Could you check a few things on this model? Use its own coordinates, in mm. Face numbers are marked on the shaded views. A direction names the side the tool comes from. Coordinates: 2 decimals unless noted, no trailing zeros. Write each loop counter-clockwise with the first axis right and the second up, starting at its lowest first coordinate (ties: lowest second). Pieces come first, ordered by that corner, then holes. Notation, with made-up numbers: M 88,20.5 L 102,20.5 A35 ccw 102,52.5 Z; hole C -32,54.25 d11. An arc over 180 degrees is marked long. Answer as CSV lines item,"result". Start each with the question number.
Item 1: If I drill on line 1 along Y through (x, z) = (31.5, -0.25); line 2 along X through (y, z) = (-2.5, 2.75); line 3 along Z through (x, y) = (22.5, 0) (3 decimals), over which ranges is the centre line in solid material (lowest first)? Write a range as [from, to].
Item 2: I'm going to push flat-ended pins straight in: P1, Ø1.5, axis at x = 23, z = 0.5, coming from the -Y side (3 decimals); P2, Ø1, axis at x = 1.5, y = 2.5, coming from the -Z side; P3, Ø2, axis at x = 3.5, z = -2, coming from the -Y side. Where does each tip first touch, or does it pass through?
Item 3: Suppose I cut it at A-A, the plane x = 2. Write out the boundary of the cut face in (y, z) (3 decimals), and give its area (3 significant figures).
Item 4: On a 3-axis mill with a long thin cutter (end or side, diameter ignored), from which of +Z, -Z, +X, -X, +Y, -Y can I reach the whole of each face in a straight line? I mean the marked faces 1, 2 and 3. Say none if no direction works.
Autodesk Inventor part; units mm, degrees
ref_plane "Work Plane1" through (29, 0, 0) normal (0, -1, 0) x (1, 0, 0)
ref_plane "YZ Plane" through (0, 0, 0) normal (1, 0, 0) x (0, 1, 0)
ref_plane "XZ Plane" through (0, 0, 0) normal (0, 1, 0) x (-1, 0, 0)
sketch "Sketch1" plane through (0, 0, 0) normal (0, 0, 1) x (1, 0, 0)
  line L0 (-1.7103, 0) -> (50.8, 0)
  line L1 (50.8, 0) -> (50.8, 3.175)
  line L2 (50.8, 3.175) -> (19.05, 3.175)
  line L3 (19.05, 3.175) -> (15.8749, 3.175)
  line L4 (15.8749, 3.175) -> (0, 3.175)
  line L5 (0, 3.175) -> (0, 4.7625)
  line L6 (0, 4.7625) -> (-6.35, 4.7625)
  line L7 (-6.35, 4.7625) -> (-6.35, 2.757)
  line L8 (-6.35, 2.757) -> (-3.302, 2.757)
  line L9 (-3.302, 2.757) -> (-1.7103, 0)
  line L10 (-16.51, 0) -> (54.61, 0)
  line L11 (0, -0.9525) -> (0, 5.715)
  line L12 (19.05, 3.175) -> (0, 3.175) construction
  dimension "d1" = 31.75
  dimension "d2" = 3.1751
  dimension "d3" = 6.35
  dimension "d4" = 3.048
  dimension "d5" = 60
  dimension "d6" = 6.35
  dimension "d7" = 6.35
  dimension "d8" = 5.5139
  dimension "d9" = 9.525
  dimension "d26" = 50.8
revolve "Body" add sketch "Sketch1" angle 360 about axis through (-1.7103, 0, 0) along (1, 0, 0)
sketch "Sketch2" plane through (-6.35, 0, 0) normal (-1, 0, 0) x (0, 0, 1)
  circle A0 centre (0, 0) radius 2.757
  line L0 (0, -6.6675) -> (0, 6.6675)
  line L1 (-6.6675, 0) -> (6.6675, 0)
  line L2 (2.757, 0) -> (1.3785, -2.3876)
  line L3 (1.3785, -2.3876) -> (-1.3785, -2.3876)
  line L4 (-1.3785, -2.3876) -> (-2.757, 0)
  line L5 (-2.757, 0) -> (-1.3785, 2.3876)
  line L6 (-1.3785, 2.3876) -> (1.3785, 2.3876)
  line L7 (1.3785, 2.3876) -> (2.757, 0)
extrude "Slot" add sketch "Sketch2" against normal up to next contours L7 A0 | A0 L2 | L6 L0 A0 | A0 L0 L3 | L0 L6 A0 | A0 L3 L0 | L4 A0 | A0 L5
fillet "Fillet1" radius 0.635 1 edges at (-6.35, -4.7625, 0)
thread "Thread"
chamfer "Chamfer1" distance 0.7556 distance2 0.7556 1 edges at (50.8, -3.175, 0) measured on face at (50.8, -0.8017, -1.6073)
ref_plane "Work Plane1" through (29, 0, 0) normal (0, -1, 0) x (1, 0, 0)
equation "\"d1\" = GEL"
equation "\"d3\" = KOH"
equation "\"d4\" = INTI"
equation "\"d6\" = GD"
equation "\"d7\" = BDM"
equation "\"d8\" = 1.1547 * SW"
equation "\"d9\" = KOD"
equation "\"d26\" = NLG"
equation "\"d17\" = RR"
equation "\"d13\" = GEL"
equation "\"d15\" = -0.5 * SPD + 0.5 * GD"
equation "\"d16\" = GUL"
equation "\"GD\" = 6.35"
equation "\"NLG\" = 50.8"
equation "\"GEL\" = 31.75"
equation "\"KOD\" = 9.525"
equation "\"KOH\" = 6.35"
equation "\"INTI\" = 3.048"
equation "\"GAL\" = 3.175"
equation "\"GUL\" = 0.75565"
equation "\"BDM\" = 6.35"
equation "\"SW\" = 4.7752"
equation "\"RR\" = 0.635"
equation "\"SPD\" = 4.8387"
equation "\"R\" = 0.1778"
equation "\"PHH\" = 0.2032"
equation "\"GD1\" = SPD"
equation "\"THREADDIA\" = 6.35"
equation "\"FAWI\" = 45deg"
equation "\"KOH1\" = 5.715"
equation "\"NND\" = 6.35"
equation "\"TOA\" = 30deg"
equation "\"E0\" = 1.155 * SW"
properties part number "am-1058" material "Steel"
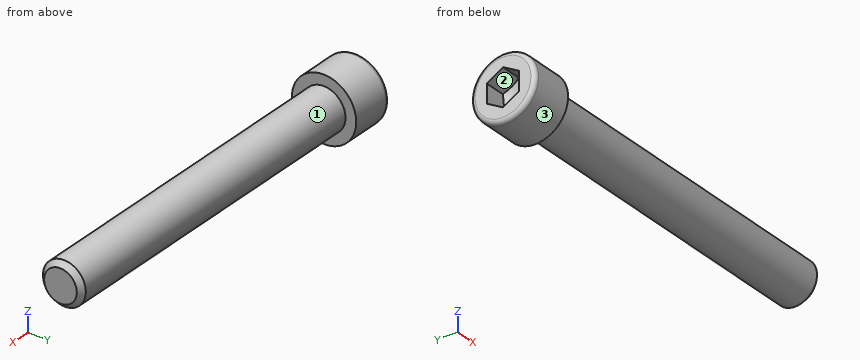
Ans:
1,line 1,"y = [-3.17, 3.17]"
1,line 2,"x = [-6.35, 0]"
1,line 3,"z = [-3.175, 3.175]"
2,P1,"stops at y = -3.175"
2,P2,"stops at z = -2.47"
2,P3,"stops at y = -3.01"
3,outline,"C 0,0 d6.35"
3,area,"31.7 mm^2"
4,face 1,"+X"
4,face 2,"-X"
4,face 3,"+X, -X"
